Could you check a few things on this model? Use its own coordinates, in mm. Face numbers are marked on the shaded views. A direction names the side the tool comes from. Round coordinates to 2 decimals unless told otherwise and drop trailing zeros. Write each loop counter-clockwise with the first axis right and the second up, starting at its lowest first coordinate (ties: lowest second). Pieces come first, ordered by that corner, then holes. Notation, with made-up numbers: (67.25, 6.25) -> (120.25, 6.25) arc R7 ccw to (120.25, 19.25) -> close; hole circle Ø2 at (42, 33). An arc over 180 degrees is marked (long way). Answer in a Markdown table with one row per item.
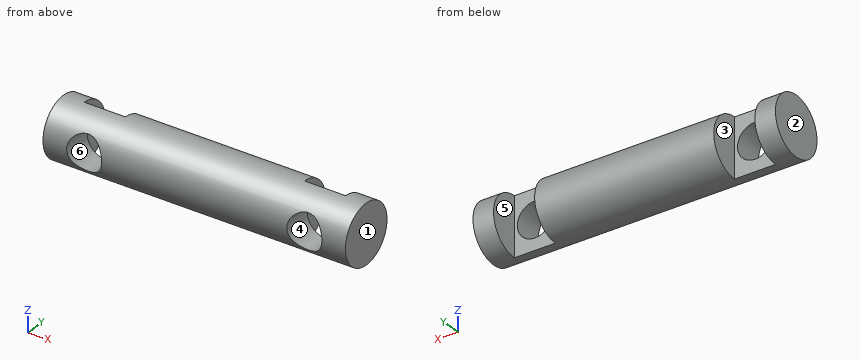
from build123d import *

# Parameters (mm, degrees)
SKETCH1_W               = 103
SKETCH1_H               = 10
CUT_EXTRUDE1_START      = -7
CUT_EXTRUDE1_DEPTH      = 14
CUT_EXTRUDE2_START      = -7
CUT_EXTRUDE2_DEPTH      = 14
CUT_EXTRUDE3_DEPTH      = 104.966340707
CUT_EXTRUDE3_DEPTH_BACK = 104.966340707
SKETCH4_R               = 5.983
SKETCH5_W               = 14
SKETCH5_H               = 25.426935298
CUT_EXTRUDE4_DEPTH      = 5


with BuildPart() as part:
    # Sketch1 → Revolve1 (revolve)
    with BuildSketch(Plane.XY, mode=Mode.PRIVATE) as revolve1_sk:
        with Locations((-51.5, 5)):
            Rectangle(SKETCH1_W, SKETCH1_H)
    revolve(revolve1_sk.sketch.rotate(Axis((-103, 0, 0), (1, 0, 0)), 90), axis=Axis((-103, 0, 0), (1, 0, 0)))

    # Sketch2 → Cut-Extrude1 (cut)
    with BuildSketch(Plane(origin=(0, 0, 0), x_dir=(0, 0, -1), z_dir=(1, 0, 0)).offset(CUT_EXTRUDE1_START)):
        with BuildLine():
            Line((-10.872335562, 5), (10.872335562, 5))
            ThreePointArc((10.872335562, 5), (0, 11.966941154), (-10.872335562, 5))
        make_face()
    extrude(amount=-CUT_EXTRUDE1_DEPTH, mode=Mode.SUBTRACT)

    # Sketch3 → Cut-Extrude2 (cut)
    with BuildSketch(Plane.ZY.offset(103).offset(CUT_EXTRUDE2_START)):
        with BuildLine():
            Line((-13.431588828, 5), (13.431588828, 5))
            ThreePointArc((13.431588828, 5), (0, 14.332047252), (-13.431588828, 5))
        make_face()
    extrude(amount=-CUT_EXTRUDE2_DEPTH, mode=Mode.SUBTRACT)

    # Sketch4 → Cut-Extrude3 (cut, two sides: drawn at the far end of the back side and taken through both)
    with BuildSketch(Plane(origin=(0, 0, 0), x_dir=(1, 0, 0), z_dir=(0, 1, 0)).offset(-CUT_EXTRUDE3_DEPTH_BACK)):
        with Locations(Location((-89, 0, 0), (0, 0, 270))):
            Circle(SKETCH4_R)
        with Locations(Location((-14, 0, 0), (0, 0, 270))):
            Circle(SKETCH4_R)
    extrude(amount=CUT_EXTRUDE3_DEPTH + CUT_EXTRUDE3_DEPTH_BACK, mode=Mode.SUBTRACT)

    # Sketch5 → Cut-Extrude4 (cut)
    with BuildSketch(Plane(origin=(0, 5, 0), x_dir=(1, 0, 0), z_dir=(0, 1, 0))):
        with Locations((-89, 0)):
            Rectangle(SKETCH5_W, SKETCH5_H)
        with Locations((-14, 0)):
            Rectangle(SKETCH5_W, SKETCH5_H)
    extrude(amount=-CUT_EXTRUDE4_DEPTH, mode=Mode.SUBTRACT)


solid = part.part
1) For the marked faces 5 and 6, which set-ups out of +Z, -Z, +X, -X, +Y, -Y let a thin tool reach every point of the face, with its end or its side?
Findings:
| item | result |
|---|---|
| face 5 | +Z, -Z, +Y |
| face 6 | +Y, -Y |
2) Thinking about a two-plate mould opening in X: for the marked faces 1, 2, 3 and 4, which applies, +X half, -X half, draft (parallel to the pull), parting line (faces both ways), or undercut?
Findings:
| item | result |
|---|---|
| face 1 | +X half |
| face 2 | -X half |
| face 3 | undercut |
| face 4 | undercut |
3) Please list where these lines run through material, in increasing order: line 1 (X direction, y = -3.5, z = 0); line 2 (X direction, y = 6.75, z = 7.25); line 3 (Z direction, x = -93.5, y = -4.5).
Findings:
| item | result |
|---|---|
| line 1 | x = -103 to -94.98, -83.02 to -19.98, -8.02 to 0 |
| line 2 | x = -103 to -96, -82 to -21, -7 to 0 |
| line 3 | z = -8.93 to -3.94, 3.94 to 8.93 |
4) Imagine slicing it at C-C, the plane y = -2. Please give me the cut outline in (x, z), plus the area to 3 significant figures.
Findings:
| item | result |
|---|---|
| outline | (-103, -9.8) -> (0, -9.8) -> (0, 9.8) -> (-103, 9.8) -> close; hole circle Ø11.97 at (-89, 0); hole circle Ø11.97 at (-14, 0) |
| area | 1,790 mm^2 |
5) Imagine slicing it at D-D, the plane x = -88. Please give me the cut outline in (y, z).
Findings:
| item | result |
|---|---|
| outline | (-8.07, -5.9) arc R10 ccw to (0, -10) -> (0, -5.9) -> close; (-8.07, 5.9) -> (0, 5.9) -> (0, 10) arc R10 ccw to start |
6) Imagine slicing it at B-B, the plane y = 2. Please give me the cut outline in (x, z).
Findings:
| item | result |
|---|---|
| outline | (-103, -9.8) -> (-96, -9.8) -> (-96, 9.8) -> (-103, 9.8) -> close; (-82, -9.8) -> (-21, -9.8) -> (-21, 9.8) -> (-82, 9.8) -> close; (-7, -9.8) -> (0, -9.8) -> (0, 9.8) -> (-7, 9.8) -> close |
7) Imagine slicing it at A-A, the plane z = 0. Please give me the cut outline in (x, y), plus the area to 3 significant figures.
Findings:
| item | result |
|---|---|
| outline | (-103, -10) -> (-94.98, -10) -> (-94.98, 0) -> (-96, 0) -> (-96, 10) -> (-103, 10) -> close; (-83.02, -10) -> (-19.98, -10) -> (-19.98, 0) -> (-21, 0) -> (-21, 10) -> (-82, 10) -> (-82, 0) -> (-83.02, 0) -> close; (-8.02, -10) -> (0, -10) -> (0, 10) -> (-7, 10) -> (-7, 0) -> (-8.02, 0) -> close |
| area | 1,540 mm^2 |
8) For pin 1 (5 mm diameter, centred on x = -16.5, z = -1.5, fed in from -Y); pin 2 (1.5 mm diameter, centred on x = -40.5, y = 4.5, fed in from +Z); pin 3 (5 mm diameter, centred on x = -62.5, y = -7.5, fed in from +Z); pin 4 (3 mm diameter, centred on x = -25.5, z = 5.5, fed in from +Y), each with a flat end and sliding along its axis, tell me the tip position at first contact or that it passes through.
Findings:
| item | result |
|---|---|
| pin 1 | passes through |
| pin 2 | stops at z = 9.27 |
| pin 3 | stops at z = 8.66 |
| pin 4 | stops at y = 9.17 |
